```python
from build123d import *

# Parameters (mm, degrees)
BOSS_EXTRUDE1_DEPTH = 10
BOSS_EXTRUDE2_DEPTH = 10
SKETCH2_R           = 2.5
CUT_EXTRUDE1_DEPTH  = 8
SKETCH3_R           = 2.5
CUT_EXTRUDE2_DEPTH  = 8


with BuildPart() as part:
    # Sketch1 → Boss-Extrude1 (new, symmetric)
    with BuildSketch(Plane(origin=(0, 0, 0), x_dir=(1, 0, 0), z_dir=(0, 1, 0))):
        Polygon((8, 8), (8, 23), (8, 33), (8, 78), (0, 78), (0, 0), (78, 0), (78, 8), (33, 8), (23, 8), align=None)
    extrude(amount=BOSS_EXTRUDE1_DEPTH, both=True)

    # Sketch1<3> → Boss-Extrude2 (add, symmetric)
    with BuildSketch(Plane(origin=(0, 0, 0), x_dir=(1, 0, 0), z_dir=(0, 1, 0))):
        Polygon((8, 33), (8, 23), (23, 8), (33, 8), align=None)
    extrude(amount=BOSS_EXTRUDE2_DEPTH, both=True)

    # Sketch2 → Cut-Extrude1 (cut)
    with BuildSketch(Plane(origin=(8, 0, 0), x_dir=(0, 0, -1), z_dir=(1, 0, 0))):
        with Locations((46, 0)):
            Circle(SKETCH2_R)
        with Locations((66, 0)):
            Circle(SKETCH2_R)
    extrude(amount=-CUT_EXTRUDE1_DEPTH, mode=Mode.SUBTRACT)

    # Sketch3 → Cut-Extrude2 (cut)
    with BuildSketch(Plane(origin=(0, 0, -8), x_dir=(-1, 0, 0), z_dir=(0, 0, -1))):
        with Locations((-66, 0)):
            Circle(SKETCH3_R)
        with Locations((-46, 0)):
            Circle(SKETCH3_R)
    extrude(amount=-CUT_EXTRUDE2_DEPTH, mode=Mode.SUBTRACT)


solid = part.part
```
For this review, take the finished solid that the model builds, in its own axes (mm). A direction names the side the tool comes from. Give positions to 0.01 mm unless a question says otherwise; leave off trailing zeros. Write each loop counter-clockwise with the first axis right and the second up, starting at its lowest first coordinate (ties: lowest second). Pieces come first, ordered by that corner, then holes.
Item 1: The part is to be moulded in two halves that separate along Y. For faces 4 (the face through (8, 0, -55)), 5 (the face through (18.6, -10, -21.8)), 6 (the face through (43.69, -0.96, -4.06)), say which applies: +Y half, -Y half, draft (parallel to the pull), parting line (faces both ways), or undercut.
Item 2: Take a section at C-C (z = -46). Give the boundary of the cut face in (x, y), and give its area (3 significant figures).
Item 3: Take a section at A-A (x = 46). Give the boundary of the cut face in (y, z), and give its area (3 significant figures).
Item 4: Insertion check: P1, Ø8, axis at y = 0, z = -46, coming from the +X side; P2, Ø10, axis at x = 38.5, y = -7.5, coming from the -Z side; P3, Ø6, axis at x = 20, y = 0, coming from the -Z side; P4, Ø3, axis at y = 0, z = -66, coming from the +X side. Each pin has a flat end and moves straight along its axis. Give the tip position at first contact, or say it passes through.
Item 5: Machinability: for faces 1 (the face through (16, 0, -8)), 2 (the face through (64.85, -2.22, -4.06)), 3 (the face through (56, 0, -8)), which of the approach directions +Z, -Z, +X, -X, +Y, -Y give a long, thin tool a straight path to every point of the face, cutting with its end or side? Answer none if there is none.
Item 6: Take a section at B-B (y = 0). Give the boundary of the cut face in (x, z).
Item 7: Wall thickness on probe 1 along Y at (x, z) = (46, -4); probe 2 along X at (y, z) = (2.25, -7.5); probe 3 along Z at (x, y) = (56, 5.75): over which ranges is each line inside the solid? List them lowest first.
Item 8: Take a section at D-D (y = -6.75). Give the boundary of the cut face in (x, z), and give its area (3 significant figures).
Established:
1. face 4: draft
1. face 5: -Y half
1. face 6: undercut
2. outline: (0, -10) - (8, -10) - (8, -2.5) - (0, -2.5) - close; (0, 2.5) - (8, 2.5) - (8, 10) - (0, 10) - close
2. area: 120 mm2
3. outline: (-10, -8) - (-2.5, -8) - (-2.5, 0) - (-10, 0) - close; (2.5, -8) - (10, -8) - (10, 0) - (2.5, 0) - close
3. area: 120 mm2
4. P1: stops at x = 8
4. P2: stops at z = -8
4. P3: stops at z = -24
4. P4: passes through
5. face 1: +Y, -Y
5. face 2: +Z, -Z
5. face 3: -Z, +X, +Y, -Y
6. outline: (0, -78) - (8, -78) - (8, -68.5) - (0, -68.5) - close; (0, -63.5) - (8, -63.5) - (8, -48.5) - (0, -48.5) - close; (0, -43.5) - (8, -43.5) - (8, -33) - (33, -8) - (43.5, -8) - (43.5, 0) - (0, 0) - close; (48.5, -8) - (63.5, -8) - (63.5, 0) - (48.5, 0) - close; (68.5, -8) - (78, -8) - (78, 0) - (68.5, 0) - close; hole (8, -23) - (23, -8) - (8, -8) - close
7. probe 1: y = -10 to -2.5, 2.5 to 10
7. probe 2: x = 0 to 44.91, 47.09 to 64.91, 67.09 to 78
7. probe 3: z = -8 to 0
8. outline: (0, -78) - (8, -78) - (8, -33) - (33, -8) - (78, -8) - (78, 0) - (0, 0) - close; hole (8, -23) - (23, -8) - (8, -8) - close
8. area: 1,380 mm2
